Part model, mm, in its own coordinate system. Give positions to 0.01 mm unless a question says otherwise; leave off trailing zeros. Answer in a Markdown table with one row per item.
from build123d import *

# Parameters (mm, degrees)
F1_DEPTH = 300


# Not quite as in the source:
# - ends of sketch curves that miss each other by under 0.0002 mm in the source are joined


with BuildPart() as f1:
    # F0 (on Top) → F1 (new body)
    with BuildSketch(Plane.XY):
        with BuildLine():
            ThreePointArc((0, 2.15), (1.5202795796, 1.5202795796), (2.15, 0))
            Line((2.15, 0), (3, 0))
            Line((3, 0), (3.307278, 0.307278))
            ThreePointArc((3.307278, 0.307278), (3.7143803747, 2.2820219924), (4.7078187099, 4.0365664363))
            ThreePointArc((4.7078187099, 4.0365664363), (4.812308461, 4.1201573706), (4.94275, 4.15))
            Line((4.94275, 4.15), (8.2, 4.15))
            ThreePointArc((8.2, 4.15), (8.4121320344, 4.0621320344), (8.5, 3.85))
            Line((8.5, 3.85), (8.5, 2.95))
            ThreePointArc((8.5, 2.95), (8.5878679656, 2.7378679656), (8.8, 2.65))
            Line((8.8, 2.65), (9.7, 2.65))
            ThreePointArc((9.7, 2.65), (9.9121320344, 2.7378679656), (10, 2.95))
            Line((10, 2.95), (10, 9.7))
            ThreePointArc((10, 9.7), (9.9121320344, 9.9121320344), (9.7, 10))
            Line((9.7, 10), (2.95, 10))
            ThreePointArc((2.95, 10), (2.7378679656, 9.9121320344), (2.65, 9.7))
            Line((2.65, 9.7), (2.65, 8.8))
            ThreePointArc((2.65, 8.8), (2.7378679656, 8.5878679656), (2.95, 8.5))
            Line((2.95, 8.5), (3.85, 8.5))
            ThreePointArc((3.85, 8.5), (4.0621320344, 8.4121320344), (4.15, 8.2))
            Line((4.15, 8.2), (4.15, 4.94275))
            ThreePointArc((4.15, 4.94275), (4.1201572004, 4.8123081084), (4.036566086, 4.7078178916))
            ThreePointArc((4.036566086, 4.7078178916), (2.2820216259, 3.7143802371), (0.3072779813, 3.3072783955))
            Line((0.3072779813, 3.3072783955), (0, 3))
            Line((0, 3), (0, 2.15))
        make_face()
        with BuildLine():
            ThreePointArc((7, 9), (8.4142135624, 8.4142135624), (9, 7))
            ThreePointArc((9, 7), (8.4142135624, 5.5857864376), (7, 5))
            ThreePointArc((7, 5), (5.5857864376, 5.5857864376), (5, 7))
            ThreePointArc((5, 7), (5.5857864376, 8.4142135624), (7, 9))
        make_face(mode=Mode.SUBTRACT)
        with BuildLine():
            Line((3, 0), (2.15, 0))
            ThreePointArc((2.15, 0), (1.5202795796, -1.5202795796), (0, -2.15))
            Line((0, -2.15), (0, -3))
            Line((0, -3), (0.307278, -3.307277))
            ThreePointArc((0.307278, -3.307277), (2.2820216259, -3.7143792371), (4.036565823, -4.7078172229))
            ThreePointArc((4.036565823, -4.7078172229), (4.1201572004, -4.8123071084), (4.15, -4.942749))
            Line((4.15, -4.942749), (4.15, -8.2))
            ThreePointArc((4.15, -8.2), (4.0621320344, -8.4121320344), (3.85, -8.5))
            Line((3.85, -8.5), (2.95, -8.5))
            ThreePointArc((2.95, -8.5), (2.7378679656, -8.5878679656), (2.65, -8.8))
            Line((2.65, -8.8), (2.65, -9.7))
            ThreePointArc((2.65, -9.7), (2.7378679656, -9.9121320344), (2.95, -10))
            Line((2.95, -10), (9.7, -10))
            ThreePointArc((9.7, -10), (9.9121320344, -9.9121320344), (10, -9.7))
            Line((10, -9.7), (10, -2.95))
            ThreePointArc((10, -2.95), (9.9121320344, -2.7378679656), (9.7, -2.65))
            Line((9.7, -2.65), (8.8, -2.65))
            ThreePointArc((8.8, -2.65), (8.5878679656, -2.7378679656), (8.5, -2.95))
            Line((8.5, -2.95), (8.5, -3.85))
            ThreePointArc((8.5, -3.85), (8.4121320344, -4.0621320344), (8.2, -4.15))
            Line((8.2, -4.15), (4.94275, -4.15))
            ThreePointArc((4.94275, -4.15), (4.8123081084, -4.1201572004), (4.7078178916, -4.036566086))
            ThreePointArc((4.7078178916, -4.036566086), (3.7143800615, -2.2820211583), (3.3072783483, -0.3072769835))
            Line((3.3072783483, -0.3072769835), (3, 0))
        make_face()
        with BuildLine():
            ThreePointArc((7, -5), (8.4142135624, -5.5857864376), (9, -7))
            ThreePointArc((9, -7), (8.4142135624, -8.4142135624), (7, -9))
            ThreePointArc((7, -9), (5.5857864376, -8.4142135624), (5, -7))
            ThreePointArc((5, -7), (5.5857864376, -5.5857864376), (7, -5))
        make_face(mode=Mode.SUBTRACT)
        with BuildLine():
            ThreePointArc((-2.15, 0), (-1.5202795796, 1.5202795796), (0, 2.15))
            Line((0, 2.15), (0, 3))
            Line((0, 3), (-0.307277, 3.307278))
            ThreePointArc((-0.307277, 3.307278), (-2.2820211583, 3.7143800615), (-4.036565823, 4.7078182229))
            ThreePointArc((-4.036565823, 4.7078182229), (-4.1201572004, 4.8123081084), (-4.15, 4.94275))
            Line((-4.15, 4.94275), (-4.15, 8.2))
            ThreePointArc((-4.15, 8.2), (-4.0621320344, 8.4121320344), (-3.85, 8.5))
            Line((-3.85, 8.5), (-2.95, 8.5))
            ThreePointArc((-2.95, 8.5), (-2.7378679656, 8.5878679656), (-2.65, 8.8))
            Line((-2.65, 8.8), (-2.65, 9.7))
            ThreePointArc((-2.65, 9.7), (-2.7378679656, 9.9121320344), (-2.95, 10))
            Line((-2.95, 10), (-9.7, 10))
            ThreePointArc((-9.7, 10), (-9.9121320344, 9.9121320344), (-10, 9.7))
            Line((-10, 9.7), (-10, 2.95))
            ThreePointArc((-10, 2.95), (-9.9121320344, 2.7378679656), (-9.7, 2.65))
            Line((-9.7, 2.65), (-8.8, 2.65))
            ThreePointArc((-8.8, 2.65), (-8.5878679656, 2.7378679656), (-8.5, 2.95))
            Line((-8.5, 2.95), (-8.5, 3.85))
            ThreePointArc((-8.5, 3.85), (-8.4121320344, 4.0621320344), (-8.2, 4.15))
            Line((-8.2, 4.15), (-4.942749, 4.15))
            ThreePointArc((-4.942749, 4.15), (-4.812307461, 4.1201573706), (-4.7078173786, 4.0365666993))
            ThreePointArc((-4.7078173786, 4.0365666993), (-3.7143793747, 2.2820219924), (-3.3072773955, 0.3072779813))
            Line((-3.3072773955, 0.3072779813), (-3, 0))
            Line((-3, 0), (-2.15, 0))
        make_face()
        with BuildLine():
            ThreePointArc((-7, 5), (-8.4142135624, 5.5857864376), (-9, 7))
            ThreePointArc((-9, 7), (-8.4142135624, 8.4142135624), (-7, 9))
            ThreePointArc((-7, 9), (-5.5857864376, 8.4142135624), (-5, 7))
            ThreePointArc((-5, 7), (-5.5857864376, 5.5857864376), (-7, 5))
        make_face(mode=Mode.SUBTRACT)
        with BuildLine():
            Line((0, -3), (0, -2.15))
            ThreePointArc((0, -2.15), (-1.5202795796, -1.5202795796), (-2.15, 0))
            Line((-2.15, 0), (-3, 0))
            Line((-3, 0), (-3.307277, -0.307277))
            ThreePointArc((-3.307277, -0.307277), (-3.7143790615, -2.2820211583), (-4.7078172229, -4.036565823))
            ThreePointArc((-4.7078172229, -4.036565823), (-4.8123071084, -4.1201572004), (-4.942749, -4.15))
            Line((-4.942749, -4.15), (-8.2, -4.15))
            ThreePointArc((-8.2, -4.15), (-8.4121320344, -4.0621320344), (-8.5, -3.85))
            Line((-8.5, -3.85), (-8.5, -2.95))
            ThreePointArc((-8.5, -2.95), (-8.5878679656, -2.7378679656), (-8.8, -2.65))
            Line((-8.8, -2.65), (-9.7, -2.65))
            ThreePointArc((-9.7, -2.65), (-9.9121320344, -2.7378679656), (-10, -2.95))
            Line((-10, -2.95), (-10, -9.7))
            ThreePointArc((-10, -9.7), (-9.9121320344, -9.9121320344), (-9.7, -10))
            Line((-9.7, -10), (-2.95, -10))
            ThreePointArc((-2.95, -10), (-2.7378679656, -9.9121320344), (-2.65, -9.7))
            Line((-2.65, -9.7), (-2.65, -8.8))
            ThreePointArc((-2.65, -8.8), (-2.7378679656, -8.5878679656), (-2.95, -8.5))
            Line((-2.95, -8.5), (-3.85, -8.5))
            ThreePointArc((-3.85, -8.5), (-4.0621320344, -8.4121320344), (-4.15, -8.2))
            Line((-4.15, -8.2), (-4.15, -4.942749))
            ThreePointArc((-4.15, -4.942749), (-4.1201572004, -4.8123071084), (-4.036566086, -4.7078168916))
            ThreePointArc((-4.036566086, -4.7078168916), (-2.2820211583, -3.7143790615), (-0.3072769835, -3.3072773483))
            Line((-0.3072769835, -3.3072773483), (0, -3))
        make_face()
        with BuildLine():
            ThreePointArc((-7, -9), (-8.4142135624, -8.4142135624), (-9, -7))
            ThreePointArc((-9, -7), (-8.4142135624, -5.5857864376), (-7, -5))
            ThreePointArc((-7, -5), (-5.5857864376, -5.5857864376), (-5, -7))
            ThreePointArc((-5, -7), (-5.5857864376, -8.4142135624), (-7, -9))
        make_face(mode=Mode.SUBTRACT)
    extrude(amount=F1_DEPTH)


solid = f1.part
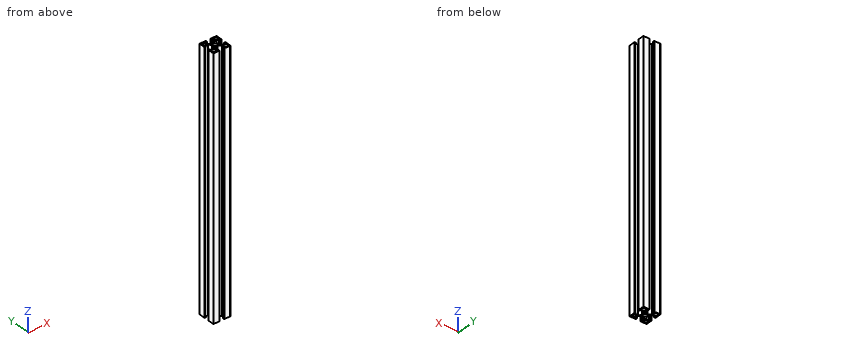
(1) Pin check, flat tip, straight feed: pin 1 Ø1 at (y, z) = (2, 88) entering from +X. Stop position of the tip, or through.
Recorded:
| item | result |
|---|---|
| pin 1 | stops at x = 3.8 |
(2) Drill centre lines: line 1 along Y through (x, z) = (7, 200); line 2 along X through (y, z) = (-4, 111); line 3 along X through (y, z) = (6, 177.5). Where is each one in solid material? Low to high.
Recorded:
| item | result |
|---|---|
| line 1 | y = -10 to -9, -5 to -4.15, 4.15 to 5, 9 to 10 |
| line 2 | x = -10 to -8.46, -4.68 to -2.93, 2.93 to 4.68, 8.46 to 10 |
| line 3 | x = -10 to -8.73, -5.27 to -4.15, 4.15 to 5.27, 8.73 to 10 |
(3) Saw through at A-A (z = 232). Give the number of separate pieces and of enclosed holes in the cut face, plus the area to 3 significant figures.
Recorded:
| item | result |
|---|---|
| separate pieces | 1 |
| enclosed holes | 5 |
| area | 146 mm^2 |
